Design review of the part shown in the three views and the two pictorial views. Dimensions are in mm from the part's minimum x, y and z. Coordinates: 2 decimals unless noted, no trailing zeros. Order: outer loops, then holes, each group sorted by start corner. A loop starts at its lowest first (then second) coordinate and runs counter-clockwise, first axis right, second up. Notation, with made-up numbers: (0.5, -37.75) -> (52.5, -37.75) arc R30 cw to (52.5, -6.75) -> close; hole circle Ø9 at (-9.75, 62). An arc over 180 degrees is marked (long way). Answer as a JSON object with one key per item and string values. Group by question number.
1) Add section D-D, the plane x = 6.75. Write out the cut boundary in (y, z).
2) For pin 1 (1.5 mm diameter, centred on y = 26.5, z = 9, fed in from -X), flat-tipped, find the tip position at first contact; note if it passes through.
3) Add section B-B, the plane y = 24. Write out the cut boundary in (x, z) (1 decimal).
4) Draft analysis for pull direction X (two halves, no side actions). For the marked faces 1, 2 and 3, state which applies: +X half, -X half, draft (parallel to the pull), parting line (faces both ways), or undercut.
5) Wall thickness on L1, parallel to X at y = 22.5, z = 11.5 (1 decimal); L2, parallel to X at y = 13.5, z = 8.5 (1 decimal); L3, parallel to Y at x = 9.25, z = 10.25: over which ranges is each line inside the solid? List them lowest first.
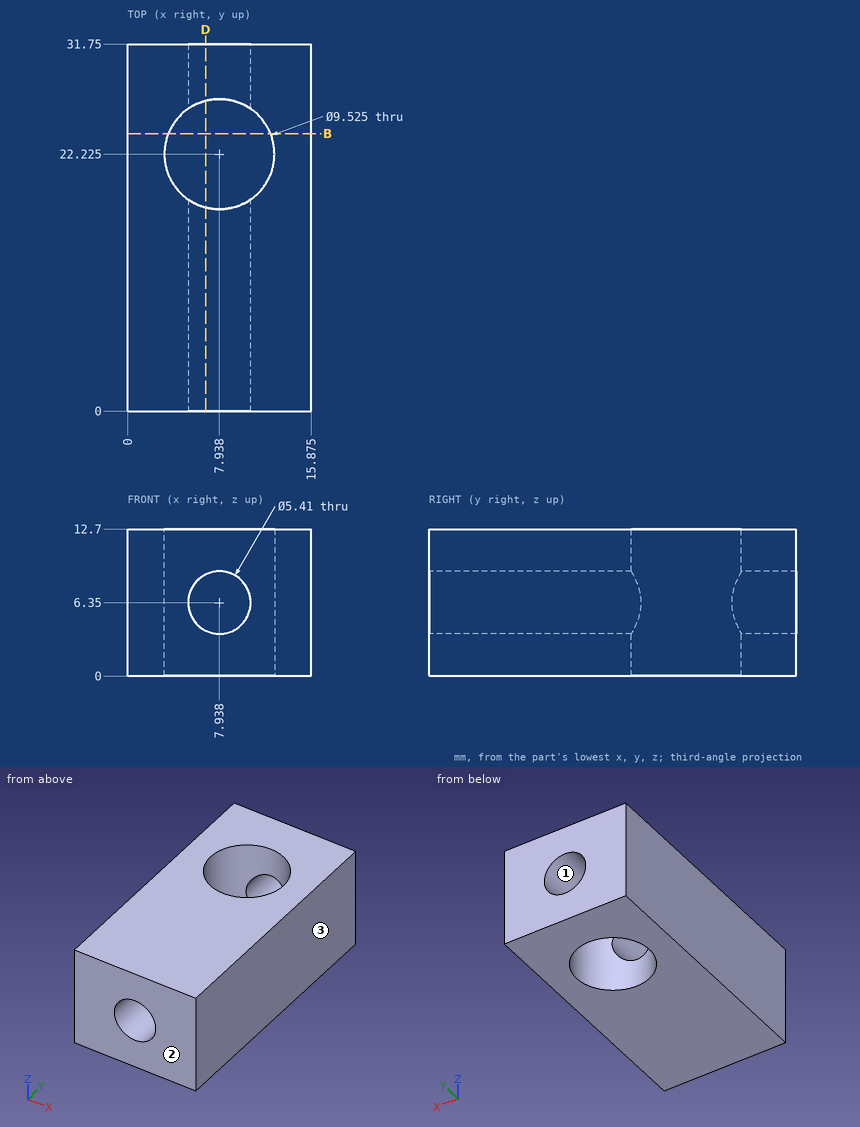
Output values:
{
 "1": {"outline": "(0, 0) -> (17.61, 0) -> (17.61, 3.92) -> (0, 3.92) -> close; (0, 8.78) -> (17.61, 8.78) -> (17.61, 12.7) -> (0, 12.7) -> close; (26.84, 0) -> (31.75, 0) -> (31.75, 3.92) -> (26.84, 3.92) -> close; (26.84, 8.78) -> (31.75, 8.78) -> (31.75, 12.7) -> (26.84, 12.7) -> close"},
 "2": {"pin 1": "stops at x = 0"},
 "3": {"outline": "(0, 0) -> (3.5, 0) -> (3.5, 12.7) -> (0, 12.7) -> close; (12.4, 0) -> (15.9, 0) -> (15.9, 12.7) -> (12.4, 12.7) -> close"},
 "4": {"face 1": "undercut", "face 2": "draft", "face 3": "+X half"},
 "5": {"L1": "x = 0 to 3.2, 12.7 to 15.9", "L2": "x = 0 to 6.3, 9.6 to 15.9", "L3": "y = 0 to 17.65, 26.8 to 31.75"}
}
